Verification items for the finished model (mm, model axes). A direction names the side the tool comes from. Round coordinates to 2 decimals unless told otherwise and drop trailing zeros. Order: outer loops, then holes, each group sorted by start corner. A loop starts at its lowest first (then second) coordinate and runs counter-clockwise, first axis right, second up. Notation, with made-up numbers: (82.25, 24.5) -> (89.25, 24.5) arc R25 cw to (89.25, 49.5) -> close; hole circle Ø1 at (60, 64.25). An arc over 180 degrees is marked (long way). Return JSON: item names as keys, results as strings. Group by question number.
Item 1: Depth check by flat-ended pin: pin 1 Ø10 at (y, z) = (-5.5, 11) entering from +X; pin 2 Ø5 at (x, z) = (2.5, 23.5) entering from -Y (3 decimals); pin 3 Ø8 at (y, z) = (4.5, 43) entering from -X. Enter the tip coordinate at first touch or a pass-through.
Item 2: Scan lines: probe 1 along Z at (x, y) = (3, 4); probe 2 along Z at (x, y) = (2, -2.75); probe 3 along Z at (x, y) = (-4.25, -4). Record each from-to range of solid material in increasing order. Write a range as from..to.
Item 3: Sectioned sample at D-D on z = 85. Record the cut outline in (x, y).
Item 4: Sectioned sample at A-A on x = 0. Record the cut outline in (y, z) (3 decimals), plus the area to 3 significant figures.
Item 5: Sectioned sample at C-C on z = 44. Record the cut outline in (x, y) (3 decimals), plus the area to 3 significant figures.
Item 6: Access from +Z, -Z, +X, -X, +Y, -Y to the whole of each face (thin tool, end or side, straight path). Record for faces 1 (the flat face through (0, 0, 100.76)), 2 (the flat face through (-4, -1, 49.69)), 3 (the cylindrical face through (5.242, -2.174, 31.874)).
```python
from build123d import *

# Parameters (mm, degrees)
SKETCH1_R           = 3.5
BOSS_EXTRUDE1_DEPTH = 14.55
SKETCH2_R           = 5.675
BOSS_EXTRUDE2_DEPTH = 35.14
SKETCH3_R           = 3.955
BOSS_EXTRUDE3_DEPTH = 5.5
SKETCH4_R           = 3
BOSS_EXTRUDE4_DEPTH = 36.6
SKETCH5_R           = 9.86
BOSS_EXTRUDE5_DEPTH = 8.97
CHAMFER1_SIZE       = 1.5


with BuildPart() as part:
    # Sketch1 → Boss-Extrude1 (new body)
    with BuildSketch(Plane.XY):
        Circle(SKETCH1_R)
    extrude(amount=BOSS_EXTRUDE1_DEPTH)

    # Sketch2 → Boss-Extrude2 (add)
    with BuildSketch(Plane.XY.offset(14.55)):
        Circle(SKETCH2_R)
    extrude(amount=BOSS_EXTRUDE2_DEPTH)

    # Sketch3 → Boss-Extrude3 (add)
    with BuildSketch(Plane.XY.offset(49.69)):
        Circle(SKETCH3_R)
    extrude(amount=BOSS_EXTRUDE3_DEPTH)

    # Sketch4 → Boss-Extrude4 (add)
    with BuildSketch(Plane.XY.offset(55.19)):
        Circle(SKETCH4_R)
    extrude(amount=BOSS_EXTRUDE4_DEPTH)

    # Sketch5 → Boss-Extrude5 (add)
    with BuildSketch(Plane.XY.offset(91.79)):
        Circle(SKETCH5_R)
    extrude(amount=BOSS_EXTRUDE5_DEPTH)

    # Chamfer1
    chamfer1_edges = [part.edges().sort_by_distance(p)[0] for p in [
        (-9.86, 0, 91.79),
        (-9.86, 0, 100.76),
    ]]
    chamfer(chamfer1_edges, length=CHAMFER1_SIZE)


solid = part.part
```
Recorded:
{
 "1": {"pin 1": "x = 5.32", "pin 2": "y = -5.675", "pin 3": "x = -5.65"},
 "2": {"probe 1": "14.55..49.69, 91.79..100.76", "probe 2": "0..55.19, 91.79..100.76", "probe 3": "91.79..100.76"},
 "3": {"outline": "circle Ø6 at (0, 0)"},
 "4": {"outline": "(-9.86, 93.29) -> (-8.36, 91.79) -> (-3, 91.79) -> (-3, 55.19) -> (-3.955, 55.19) -> (-3.955, 49.69) -> (-5.675, 49.69) -> (-5.675, 14.55) -> (-3.5, 14.55) -> (-3.5, 0) -> (3.5, 0) -> (3.5, 14.55) -> (5.675, 14.55) -> (5.675, 49.69) -> (3.955, 49.69) -> (3.955, 55.19) -> (3, 55.19) -> (3, 91.79) -> (8.36, 91.79) -> (9.86, 93.29) -> (9.86, 99.26) -> (8.36, 100.76) -> (-8.36, 100.76) -> (-9.86, 99.26) -> close", "area": "936 mm²"},
 "5": {"outline": "circle Ø11.35 at (0, 0)", "area": "101 mm²"},
 "6": {"face 1": "+Z, +X, -X, +Y, -Y", "face 2": "none", "face 3": "-Z"}
}
